CAD build for the part. Positions are in the model's coordinates, mm. Face numbers are marked on the shaded views. A direction names the side the tool comes from. Coordinates: 2 decimals unless noted, no trailing zeros. Loops run counter-clockwise (first coordinate to the right, second up) from the corner with the lowest first, then second, coordinate; pieces in that order, holes last. Notation, with made-up numbers: (18.5, -31) -> (28.5, -31) arc R19 ccw to (28.5, 3) -> close; hole circle Ø7 at (-18.75, 76.5). An arc over 180 degrees is marked (long way). Answer as a JSON object with one key per item and string values. Group by question number.
from build123d import *

# Parameters (mm, degrees)
BOSS_EXTRUDE1_DEPTH          = 25
CUT_EXTRUDE_THIN1_DEPTH      = 40.986996748
CUT_EXTRUDE_THIN1_DEPTH_BACK = 8.5
CUT_EXTRUDE_THIN3_DEPTH      = 40.986996748
CUT_EXTRUDE_THIN3_DEPTH_BACK = 8.5
SKETCH5_W                    = 32
SKETCH5_H                    = 19.425554826
BOSS_EXTRUDE2_DEPTH          = 3
CHAMFER3_SIZE                = 3
CHAMFER4_SIZE                = 1


with BuildPart() as part:
    # Sketch2 → Boss-Extrude1 (new body)
    with BuildSketch(Plane(origin=(0, 0, 0), x_dir=(1, 0, 0), z_dir=(0, 1, 0))):
        Polygon((0, 0), (0, 13.5), (2.962777413, 16.462777413), (21.462777413, 16.462777413), (24.425554826, 13.5), (24.425554826, 0), (21.462777413, -2.962777413), (2.962777413, -2.962777413), align=None)
    extrude(amount=BOSS_EXTRUDE1_DEPTH)

    # Sketch3 → Cut-Extrude-Thin1 (cut, two sides: drawn at the far end of the back side and taken through both)
    with BuildSketch(Plane.XY.offset(2.962777413).offset(-CUT_EXTRUDE_THIN1_DEPTH_BACK)):
        with BuildLine():
            Line((6.962777413, 0), (6.962777413, 20))
            ThreePointArc((6.962777413, 20), (8.712777413, 21.75), (10.462777413, 20))
            Line((10.462777413, 20), (10.462777413, 16.688890745))
            Line((10.462777413, 16.688890745), (18.462777413, 16.688890745))
            Line((18.462777413, 16.688890745), (18.462777413, 15.188890745))
            Line((18.462777413, 15.188890745), (10.462777413, 15.188890745))
            Line((10.462777413, 15.188890745), (10.462777413, 10.688890745))
            Line((10.462777413, 10.688890745), (18.462777413, 10.688890745))
            Line((18.462777413, 10.688890745), (18.462777413, 9.188890745))
            Line((18.462777413, 9.188890745), (10.462777413, 9.188890745))
            Line((10.462777413, 9.188890745), (10.462777413, 0))
            Line((10.462777413, 0), (11.962777413, 0))
            Line((11.962777413, 0), (11.962777413, 7.688890745))
            Line((11.962777413, 7.688890745), (19.962777413, 7.688890745))
            Line((19.962777413, 7.688890745), (19.962777413, 12.188890745))
            Line((19.962777413, 12.188890745), (11.962777413, 12.188890745))
            Line((11.962777413, 12.188890745), (11.962777413, 13.688890745))
            Line((11.962777413, 13.688890745), (19.962777413, 13.688890745))
            Line((19.962777413, 13.688890745), (19.962777413, 18.188890745))
            Line((19.962777413, 18.188890745), (11.962777413, 18.188890745))
            Line((11.962777413, 18.188890745), (11.962777413, 20))
            ThreePointArc((11.962777413, 20), (8.712777413, 23.25), (5.462777413, 20))
            Line((5.462777413, 20), (5.462777413, 0))
            Line((5.462777413, 0), (6.962777413, 0))
        make_face()
    extrude(amount=CUT_EXTRUDE_THIN1_DEPTH + CUT_EXTRUDE_THIN1_DEPTH_BACK, mode=Mode.SUBTRACT)

    # Sketch4 → Cut-Extrude-Thin3 (cut, two sides: drawn at the far end of the back side and taken through both)
    with BuildSketch(Plane(origin=(0, 0, -16.462777413), x_dir=(-1, 0, 0), z_dir=(0, 0, -1)).offset(-CUT_EXTRUDE_THIN3_DEPTH_BACK)):
        with BuildLine():
            Line((-17.462777413, 0), (-17.462777413, 19.789881458))
            ThreePointArc((-17.462777413, 19.789881458), (-15.712777413, 21.539881458), (-13.962777413, 19.789881458))
            Line((-13.962777413, 19.789881458), (-13.962777413, 16.039881458))
            Line((-13.962777413, 16.039881458), (-5.962777413, 16.039881458))
            Line((-5.962777413, 16.039881458), (-5.962777413, 14.539881458))
            Line((-5.962777413, 14.539881458), (-13.962777413, 14.539881458))
            Line((-13.962777413, 14.539881458), (-13.962777413, 10.039881458))
            Line((-13.962777413, 10.039881458), (-5.962777413, 10.039881458))
            Line((-5.962777413, 10.039881458), (-5.962777413, 8.539881458))
            Line((-5.962777413, 8.539881458), (-13.962777413, 8.539881458))
            Line((-13.962777413, 8.539881458), (-13.962777413, 0))
            Line((-13.962777413, 0), (-12.462777413, 0))
            Line((-12.462777413, 0), (-12.462777413, 7.039881458))
            Line((-12.462777413, 7.039881458), (-4.462777413, 7.039881458))
            Line((-4.462777413, 7.039881458), (-4.462777413, 11.539881458))
            Line((-4.462777413, 11.539881458), (-12.462777413, 11.539881458))
            Line((-12.462777413, 11.539881458), (-12.462777413, 13.039881458))
            Line((-12.462777413, 13.039881458), (-4.462777413, 13.039881458))
            Line((-4.462777413, 13.039881458), (-4.462777413, 17.539881458))
            Line((-4.462777413, 17.539881458), (-12.462777413, 17.539881458))
            Line((-12.462777413, 17.539881458), (-12.462777413, 19.789881458))
            ThreePointArc((-12.462777413, 19.789881458), (-15.712777413, 23.039881458), (-18.962777413, 19.789881458))
            Line((-18.962777413, 19.789881458), (-18.962777413, 0))
            Line((-18.962777413, 0), (-17.462777413, 0))
        make_face()
    extrude(amount=CUT_EXTRUDE_THIN3_DEPTH + CUT_EXTRUDE_THIN3_DEPTH_BACK, mode=Mode.SUBTRACT)

    # Sketch5 → Boss-Extrude2 (add)
    with BuildSketch(Plane(origin=(0, 25, 0), x_dir=(1, 0, 0), z_dir=(0, 1, 0))):
        with Locations((12.212777413, 6.75)):
            Rectangle(SKETCH5_W, SKETCH5_H)
    extrude(amount=BOSS_EXTRUDE2_DEPTH)

    # Chamfer3
    chamfer3_edges = [part.edges().sort_by_distance(p)[0] for p in [
        (28.212777413, 26.5, 2.962777413),
        (28.212777413, 26.5, -16.462777413),
        (-3.787222587, 26.5, -16.462777413),
        (-3.787222587, 26.5, 2.962777413),
    ]]
    chamfer(chamfer3_edges, length=CHAMFER3_SIZE)

    # Chamfer4
    chamfer4_edges = [part.edges().sort_by_distance(p)[0] for p in [
        (13.962777413, 8.539881458, -12.212777413),
        (4.462777413, 7.039881458, -12.212777413),
        (4.462777413, 11.539881458, -12.212777413),
        (4.462777413, 13.039881458, -12.212777413),
        (4.462777413, 17.539881458, -12.212777413),
        (13.962777413, 16.039881458, -12.212777413),
        (13.962777413, 14.539881458, -12.212777413),
        (13.962777413, 10.039881458, -12.212777413),
        (19.962777413, 7.688890745, -1.287222587),
        (19.962777413, 12.188890745, -1.287222587),
        (19.962777413, 13.688890745, -1.287222587),
        (19.962777413, 18.188890745, -1.287222587),
        (10.462777413, 16.688890745, -1.287222587),
        (10.462777413, 15.188890745, -1.287222587),
        (10.462777413, 10.688890745, -1.287222587),
        (10.462777413, 9.188890745, -1.287222587),
    ]]
    chamfer(chamfer4_edges, length=CHAMFER4_SIZE)


solid = part.part
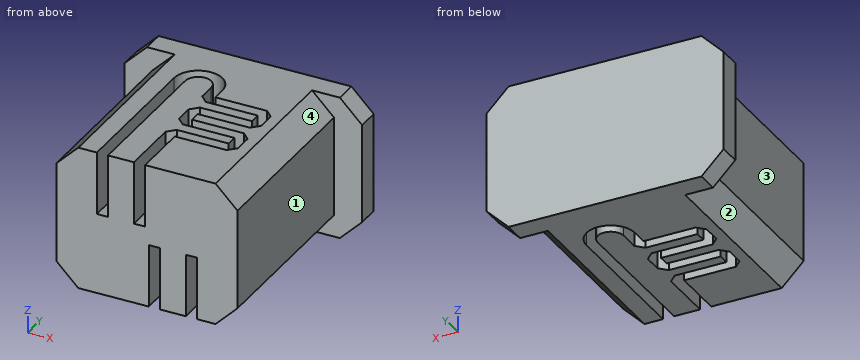
Item 1: Band-saw the part on C-C, the plane x = 26. List the corners of the cut face in (y, z).
Item 2: 3-axis set-ups, long thin cutter, end or side, ignore diameter. For the marked faces 1, 2, 3 and 4: which of +Z, -Z, +X, -X, +Y, -Y reach the whole face in a straight line?
Item 3: Drill centre lines: L1, parallel to X at y = 15.25, z = -4; L2, parallel to X at y = 19.75, z = -2.5; L3, parallel to Y at x = 13, z = -5.5. Where is each one in solid material? Low to high.
Item 4: Band-saw the part on A-A, the plane y = 25.5. List the corners of the cut face in (x, z), and give its area (3 significant figures).
Item 5: Flat gauge pins, fed straight in: P1, Ø7, axis at y = 10.5, z = -4, coming from the -X side; P2, Ø1.2, axis at y = 13.5, z = -2.5, coming from the +X side; P3, Ø6, axis at x = 24.5, y = 16.5, coming from the +Z side. Where does each tip first touch, or does it go through?
Reply:
{
 "1": {"outline": "(25, -15.68) -> (28, -15.68) -> (28, 2.18) -> (25, 2.18) -> close"},
 "2": {"face 1": "+Z, -Z, +X, -Y", "face 2": "-Z, -X, -Y", "face 3": "+Z, -Z, -X, -Y", "face 4": "+Z, +X, -Y"},
 "3": {"L1": "0 to 5.46, 6.96 to 18.46, 19.96 to 24.43", "L2": "0 to 5.46, 6.96 to 10.46, 11.96 to 24.43", "L3": "0 to 7.69, 9.19 to 10.69, 12.19 to 13.69, 15.19 to 16.69, 18.19 to 28"},
 "4": {"outline": "(-3.79, -13.46) -> (-0.79, -16.46) -> (25.21, -16.46) -> (28.21, -13.46) -> (28.21, -0.04) -> (25.21, 2.96) -> (-0.79, 2.96) -> (-3.79, -0.04) -> close", "area": "604 mm²"},
 "5": {"P1": "x = 0", "P2": "x = 24.43", "P3": "z = 2.93"}
}
